from build123d import *

# Parameters (mm, degrees)
CROQUIS1_R              = 2.5
SALIENTE_EXTRUIR1_DEPTH = 14
CROQUIS2_R              = 4.5
SALIENTE_EXTRUIR2_DEPTH = 2.5
CROQUIS3_R              = 1
CORTAR_EXTRUIR1_DEPTH   = 3


with BuildPart() as part:
    # Croquis1 → Saliente-Extruir1 (new body)
    with BuildSketch(Plane(origin=(0, 0, 0), x_dir=(1, 0, 0), z_dir=(0, 1, 0))):
        with Locations(Location((0, 0, 0), (0, 0, 270))):
            Circle(CROQUIS1_R)
    extrude(amount=SALIENTE_EXTRUIR1_DEPTH)

    # Croquis2 → Saliente-Extruir2 (add)
    with BuildSketch(Plane(origin=(0, 14, 0), x_dir=(1, 0, 0), z_dir=(0, 1, 0))):
        with Locations(Location((0, 0, 0), (0, 0, 270))):
            Circle(CROQUIS2_R)
    extrude(amount=SALIENTE_EXTRUIR2_DEPTH)

    # Croquis3 → Cortar-Extruir1 (cut, symmetric)
    with BuildSketch(Plane.XY):
        with Locations(Location((0, 10, 0), (0, 0, 89.999999999))):
            Circle(CROQUIS3_R)
    extrude(amount=CORTAR_EXTRUIR1_DEPTH, both=True, mode=Mode.SUBTRACT)


solid = part.part
For this review, take the finished solid that the model builds, in its own axes (mm). A direction names the side the tool comes from. Coordinates: 2 decimals unless noted, no trailing zeros. Order: outer loops, then holes, each group sorted by start corner. A loop starts at its lowest first (then second) coordinate and runs counter-clockwise, first axis right, second up. Notation, with made-up numbers: (75.25, 68) - (90.25, 68) arc R27 ccw to (90.25, 91) - close; hole circle Ø10 at (-18, 52). An arc over 180 degrees is marked (long way). Answer as CSV lines item,"result". Start each with the question number.
1) Add section B-B (z = 0). State the section outline as (x, y) points.
2) Add section C-C (y = 14.5). State the section outline as (x, z) points.
3) To check wall thickness, follow line 1 along Y through (x, z) = (2.5, 0.5); line 2 along X through (y, z) = (10, 0.8); line 3 along Y through (x, z) = (0.25, 1.25). State the ranges of each line that lie inside material, in increasing order. Write a range as [from, to].
4) Draft analysis for pull direction Y (two halves, no side actions). For faces 3 (the cylindrical face through (0, 9, 0)), 4 (the flat face through (0, 16.5, 0)), 5 (the cylindrical face through (1.352, 15.232, 4.292)), state which applies: +Y half, -Y half, draft (parallel to the pull), parting line (faces both ways), or undercut.
5) Add section D-D (x = 1.75). State the section outline as (y, z) points, then the cut area to 3 significant figures.
6) Machinability: for faces 1 (the cylindrical face through (0.1, 6.9, -2.5)), 2 (the flat face through (0, 0, 0)), which of the approach directions +Z, -Z, +X, -X, +Y, -Y give a long, thin tool a straight path to every point of the face, cutting with its end or side? Answer none if there is none.
7) Insertion check: P1, Ø3, axis at x = 3.5, y = 4.5, coming from the -Z side; P2, Ø2.5, axis at x = 1, z = -0.5, coming from the -Y side; P3, Ø1, axis at y = 14.5, z = 1, coming from the +X side. Each pin has a flat end and moves straight along its axis. Give the tip position at first contact, or say it passes through.
8) Add section A-A (x = 0). State the section outline as (y, z) points, then the cut area to 3 significant figures.
Result:
1,outline,"(-4.5, 14) - (-2.5, 14) - (-2.5, 0) - (2.5, 0) - (2.5, 14) - (4.5, 14) - (4.5, 16.5) - (-4.5, 16.5) - close; hole circle Ø2 at (0, 10)"
2,outline,"circle Ø9 at (0, 0)"
3,line 1,"[14, 16.5]"
3,line 2,"[-2.37, -1], [1, 2.37]"
3,line 3,"[0, 9.03], [10.97, 16.5]"
4,face 3,"undercut"
4,face 4,"+Y half"
4,face 5,"draft"
5,outline,"(0, -1.79) - (14, -1.79) - (14, -4.15) - (16.5, -4.15) - (16.5, 4.15) - (14, 4.15) - (14, 1.79) - (0, 1.79) - close"
5,area,"70.7 mm^2"
6,face 1,"-Y"
6,face 2,"+Z, -Z, +X, -X, -Y"
7,P1,"z = -1.5"
7,P2,"y = 0"
7,P3,"x = 4.47"
8,outline,"(0, -2.5) - (9, -2.5) - (9, 2.5) - (0, 2.5) - close; (11, -2.5) - (14, -2.5) - (14, -4.5) - (16.5, -4.5) - (16.5, 4.5) - (14, 4.5) - (14, 2.5) - (11, 2.5) - close"
8,area,"82.5 mm^2"
